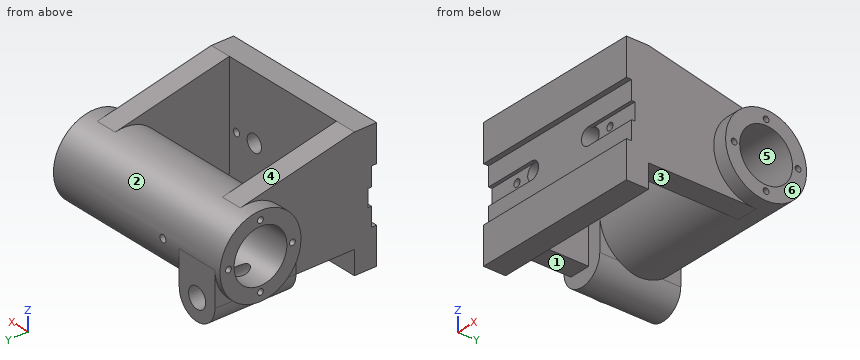
from build123d import *

# Parameters (mm, degrees)
SKETCH_2_R                   = 47.5
EXTRUDE_1_DEPTH              = 233
EXTRUDE_2_DEPTH              = 47.5
SKETCH_6_W                   = 200
SKETCH_6_H                   = 150
EXTRUDE_3_DEPTH              = 26
CUT_EXTRUDE_2_DEPTH          = 274.856257996
CUT_EXTRUDE_2_DEPTH_BACK     = 274.856257996
SKETCH_7_W                   = 64
SKETCH_7_H                   = 12
SKETCH_9_R                   = 10
CUT_EXTRUDE_3_DEPTH          = 20
SKETCH_11_W                  = 4.25
SKETCH_11_H                  = 20.001
HOLE_WIZARD_M10_1_AT_2_COUNT = 2
HOLE_WIZARD_M10_1_AT_2_PITCH = 130
CUT_EXTRUDE_START            = -60
SKETCH_12_W                  = 20
SKETCH_12_H                  = 8
CUT_EXTRUDE_4_DEPTH          = 60
EXTRUDE_6_DEPTH              = 25
RIB_8_REACH                  = 275.856
SKETCH_18_WALL_W             = 686.623983736
SKETCH_18_WALL_H             = 25
EXTRUDE_START                = -25
EXTRUDE_7_DEPTH              = 25
SKETCH_20_W                  = 25
SKETCH_20_H                  = 47.5
EXTRUDE_10_DEPTH             = 50
CUT_EXTRUDE_1_DEPTH          = 288.078386589
CUT_EXTRUDE_1_DEPTH_BACK     = 288.078386589
SKETCH_3_R                   = 31
HOLE_WIZARD_M8_1_AT_2_COUNT  = 2
HOLE_WIZARD_M8_1_AT_2_PITCH  = 53.033008589
HOLE_WIZARD_M8_1_AT_3_COUNT  = 2
HOLE_WIZARD_M8_1_AT_3_PITCH  = 75
HOLE_WIZARD_M8_1_AT_4_COUNT  = 2
HOLE_WIZARD_M8_1_AT_4_PITCH  = 53.033008589
SKETCH_27_W                  = 4.25
SKETCH_27_H                  = 47.5
SKETCH_16_R                  = 12
CUT_EXTRUDE_6_DEPTH          = 85


with BuildPart() as part:
    # Sketch 2 → Extrude 1 (new body)
    with BuildSketch(Plane(origin=(0, 0, 0), x_dir=(0, 0, -1), z_dir=(1, 0, 0))):
        Circle(SKETCH_2_R)
    extrude(amount=EXTRUDE_1_DEPTH)

    # Sketch 4 → Extrude 2 (add, symmetric)
    with BuildSketch(Plane(origin=(0, 0, 0), x_dir=(1, 0, 0), z_dir=(0, 1, 0))):
        with BuildLine():
            Line((7, 40), (7, 0))
            Line((7, 0), (57, 0))
            Line((57, 0), (57, 40))
            ThreePointArc((57, 40), (32, 65), (7, 40))
        make_face()
    extrude(amount=EXTRUDE_2_DEPTH, both=True)



with BuildPart() as body_2:
    # Sketch 6 → Extrude 3 (new body)
    with BuildSketch(Plane(origin=(0, -150, 0), x_dir=(1, 0, 0), z_dir=(0, 1, 0))):
        with Locations((116.5, 0)):
            Rectangle(SKETCH_6_W, SKETCH_6_H)
    extrude(amount=EXTRUDE_3_DEPTH)

    # Sketch 7 → Cut-Extrude 2 (cut, two sides: drawn at the far end of the back side and taken through both)
    with BuildSketch(Plane.ZY.offset(-16.5).offset(-CUT_EXTRUDE_2_DEPTH_BACK)):
        with Locations((0, -150)):
            Rectangle(SKETCH_7_W, SKETCH_7_H)
    extrude(amount=CUT_EXTRUDE_2_DEPTH + CUT_EXTRUDE_2_DEPTH_BACK, mode=Mode.SUBTRACT)

    # Sketch 9 → Cut-Extrude 3 (cut)
    with BuildSketch(Plane(origin=(0, -124, 0), x_dir=(1, 0, 0), z_dir=(0, 1, 0))):
        with Locations(Location((76.5, 0, 0), (0, 0, 270))):
            Circle(SKETCH_9_R)
        with Locations(Location((156.5, 0, 0), (0, 0, 270))):
            Circle(SKETCH_9_R)
    extrude(amount=-CUT_EXTRUDE_3_DEPTH, mode=Mode.SUBTRACT)

    # Sketch 11 → Hole Wizard M10 _1 (revolve, cut)
    with BuildSketch(Plane(origin=(181.5, -124, 0), x_dir=(0, 0, 1), z_dir=(1, 0, 0))):
        with Locations((2.125, 10.0005)):
            Rectangle(SKETCH_11_W, SKETCH_11_H)
    hole_wizard_m10_1 = revolve(axis=Axis((181.5, -117.65, 0), (0, -1, 0)), mode=Mode.SUBTRACT)

    # Hole Wizard M10 _1 at 2: Hole Wizard M10 _1 ×2
    with Locations(*[(-i * HOLE_WIZARD_M10_1_AT_2_PITCH, 0, 0) for i in range(1, HOLE_WIZARD_M10_1_AT_2_COUNT)]):
        add(hole_wizard_m10_1, mode=Mode.SUBTRACT)

    # Sketch 12 → Cut-Extrude 4 (cut)
    with BuildSketch(Plane.ZY.offset(-16.5).offset(CUT_EXTRUDE_START)):
        with Locations((0, -144)):
            Rectangle(SKETCH_12_W, SKETCH_12_H)
    cut_extrude_4 = extrude(amount=CUT_EXTRUDE_4_DEPTH, mode=Mode.SUBTRACT)

    # Mirror 1: Cut-Extrude 4 across plane
    add(cut_extrude_4.mirror(Plane.ZY.offset(-116.5)), mode=Mode.SUBTRACT)


with BuildPart() as part_1:
    add(part.part)

    add(body_2.part)  # Extrude 6 merges body 2
    # Sketch 13 → Extrude 6 (add)
    with BuildSketch(Plane.ZY.offset(-16.5)):
        with BuildLine():
            Line((-47.5, -124), (-35, -124))
            Line((-35, -124), (-35, -82.5))
            ThreePointArc((-35, -82.5), (-24.748737342, -57.751262658), (0, -47.5))
            Line((0, -47.5), (-47.5, -47.5))
            Line((-47.5, -47.5), (-47.5, -124))
        make_face()
    extrude(amount=-EXTRUDE_6_DEPTH)

    # Sketch 18 wall → Rib 8 (add, up to next)
    with BuildSketch(Plane(origin=(16.5, -57.048519027, 60.728115209), x_dir=(0, 0.978025903544, -0.208483409404), z_dir=(0, -0.208483409404, -0.978025903544)), mode=Mode.PRIVATE) as rib_8_sk1:
        with Locations((0, 12.5)):
            Rectangle(SKETCH_18_WALL_W, SKETCH_18_WALL_H)
    rib_8_tool1 = extrude(rib_8_sk1.sketch, amount=RIB_8_REACH, mode=Mode.PRIVATE) - part_1.part
    add(rib_8_tool1.solids().sort_by_distance((16.5, -57.048519027, 60.728115209))[0])

    # Sketch 19 → Extrude 7 (add)
    with BuildSketch(Plane(origin=(216.5, 0, 0), x_dir=(0, 0, -1), z_dir=(1, 0, 0)).offset(EXTRUDE_START)):
        with BuildLine():
            Line((47.5, -47.5), (0, -47.5))
            ThreePointArc((0, -47.5), (-36.92316815, -29.881928548), (-46.456230418, 9.902961947))
            Line((-46.456230418, 9.902961947), (-75, -124))
            Line((-75, -124), (47.5, -124))
            Line((47.5, -124), (47.5, -47.5))
        make_face()
    extrude(amount=EXTRUDE_7_DEPTH)

    # Sketch 20 → Extrude 10 (add)
    with BuildSketch(Plane(origin=(0, -47.5, 0), x_dir=(1, 0, 0), z_dir=(0, 1, 0))):
        with Locations((204, 23.75)):
            Rectangle(SKETCH_20_W, SKETCH_20_H)
    extrude(amount=EXTRUDE_10_DEPTH)

    # Sketch 3 → Cut-Extrude 1 (cut, two sides: drawn at the far end of the back side and taken through both)
    with BuildSketch(Plane.ZY.offset(-CUT_EXTRUDE_1_DEPTH_BACK)):
        Circle(SKETCH_3_R)
    extrude(amount=CUT_EXTRUDE_1_DEPTH + CUT_EXTRUDE_1_DEPTH_BACK, mode=Mode.SUBTRACT)

    # Sketch 25 → Hole Wizard M8 _1 (revolve, cut)
    with BuildSketch(Plane(origin=(0, 0, -37.5), x_dir=(0, 0, 1), z_dir=(0, 1, 0))):
        Polygon((0, 0), (0, 23), (3.4, 20.957073895), (3.4, 0), align=None)
    hole_wizard_m8_1 = revolve(axis=Axis((-6.35, 0, -37.5), (1, 0, 0)), mode=Mode.SUBTRACT)

    # Hole Wizard M8 _1 at 2: Hole Wizard M8 _1 ×2
    with Locations(*[Vector(0, 0.7071067811865476, 0.7071067811865476) * (i * HOLE_WIZARD_M8_1_AT_2_PITCH) for i in range(1, HOLE_WIZARD_M8_1_AT_2_COUNT)]):
        add(hole_wizard_m8_1, mode=Mode.SUBTRACT)

    # Hole Wizard M8 _1 at 3: Hole Wizard M8 _1 ×2
    with Locations(*[(0, 0, i * HOLE_WIZARD_M8_1_AT_3_PITCH) for i in range(1, HOLE_WIZARD_M8_1_AT_3_COUNT)]):
        add(hole_wizard_m8_1, mode=Mode.SUBTRACT)

    # Hole Wizard M8 _1 at 4: Hole Wizard M8 _1 ×2
    with Locations(*[Vector(0, -0.7071067811865476, 0.7071067811865476) * (i * HOLE_WIZARD_M8_1_AT_4_PITCH) for i in range(1, HOLE_WIZARD_M8_1_AT_4_COUNT)]):
        add(hole_wizard_m8_1, mode=Mode.SUBTRACT)

    # Mirror 6: Hole Wizard M8 _1 across plane
    add(hole_wizard_m8_1.mirror(Plane.ZY.offset(-116.5)), mode=Mode.SUBTRACT)

    # Mirror 6 copy 1 sketch → Mirror 6 copy 1 (revolve, cut)
    with BuildSketch(Plane(origin=(233, 37.5, 0), x_dir=(0, 0, 1), z_dir=(0, 1, 0))):
        Polygon((0, 0), (0, -23), (3.4, -20.957073895), (3.4, 0), align=None)
    revolve(axis=Axis((239.35, 37.5, 0), (1, 0, 0)), mode=Mode.SUBTRACT)

    # Mirror 6 copy 2 sketch → Mirror 6 copy 2 (revolve, cut)
    with BuildSketch(Plane(origin=(233, 0, 37.5), x_dir=(0, 0, 1), z_dir=(0, 1, 0))):
        Polygon((0, 0), (0, -23), (3.4, -20.957073895), (3.4, 0), align=None)
    revolve(axis=Axis((239.35, 0, 37.5), (1, 0, 0)), mode=Mode.SUBTRACT)

    # Mirror 6 copy 3 sketch → Mirror 6 copy 3 (revolve, cut)
    with BuildSketch(Plane(origin=(233, -37.5, 0), x_dir=(0, 0, 1), z_dir=(0, 1, 0))):
        Polygon((0, 0), (0, -23), (3.4, -20.957073895), (3.4, 0), align=None)
    revolve(axis=Axis((239.35, -37.5, 0), (1, 0, 0)), mode=Mode.SUBTRACT)

    # Sketch 27 → Hole Wizard M10 _1 2 (revolve, cut)
    with BuildSketch(Plane(origin=(80, 0, 0), x_dir=(0, 0, -1), z_dir=(1, 0, 0))):
        with Locations((2.125, 23.75)):
            Rectangle(SKETCH_27_W, SKETCH_27_H)
    revolve(axis=Axis((80, -6.35, 0), (0, 1, 0)), mode=Mode.SUBTRACT)

    # Sketch 16 → Cut-Extrude 6 (cut)
    with BuildSketch(Plane(origin=(0, 47.5, 0), x_dir=(1, 0, 0), z_dir=(0, 1, 0))):
        with Locations(Location((32, 40, 0), (0, 0, 270))):
            Circle(SKETCH_16_R)
    extrude(amount=-CUT_EXTRUDE_6_DEPTH, mode=Mode.SUBTRACT)


solid = part_1.part
Check sheet for the modelled part. Datum: model origin and axes. Units: mm. Face numbers are marked on the shaded views. A direction names the side the tool comes from. Round coordinates to 2 decimals unless told otherwise and drop trailing zeros. Write each loop counter-clockwise with the first axis right and the second up, starting at its lowest first coordinate (ties: lowest second). Pieces come first, ordered by that corner, then holes. Notation, with made-up numbers: (30.5, 39.5) -> (66.5, 39.5) arc R14 cw to (66.5, 60.5) -> close; hole circle Ø3 at (27.5, -19.5). An arc over 180 degrees is marked (long way). Answer as CSV lines item,"result". Start each with the question number.
1) Go/stop test with flat-tipped pins: P1, Ø6, axis at x = 129.5, z = -42, coming from the +Y side; P2, Ø5, axis at y = -88.5, z = 36, coming from the +X side; P3, Ø4, axis at x = 208.5, y = -5.5, coming from the +Z side; P4, Ø5, axis at y = -23, z = 58, coming from the +X side. Record where each tip stops, or that it passes through.
2) Section check C-C on x = 195.5. Enter the section's corners in (y, z), and give its area (3 significant figures).
3) Section check B-B on z = -55. Enter the section's corners in (x, y), and give its area (3 significant figures).
4) Tool access check on the marked faces 1, 2 and 3. Record the directions out of +Z, -Z, +X, -X, +Y, -Y that give a thin tool (end or side, any length) a straight path to the whole face; none if there is none.
5) Section check D-D on y = -109.5. Enter the section's corners in (x, z).
6) Release check for a two-part mould opening along Z. For the marked faces 4, 5 and 6 record: pulls with the +Z half, pulls with the -Z half, needs draft (parallel to the pull), parting line crosses it, or undercut.
7) Section check A-A on x = 125. Enter the section's corners in (y, z), and give its area (3 significant figures).
8) Material ranges on line 1 (X direction, y = -129, z = 0); line 2 (Y direction, x = 99, z = -1.5); line 3 (X direction, y = -109, z = -38), recorded low to high. Write a range as from..to.
Found:
1,P1,"stops at y = 27.12"
1,P2,"stops at x = 216.5"
1,P3,"stops at z = 50.17"
1,P4,"passes through"
2,outline,"(-150, -75) -> (-124, -75) -> (-124, -47.5) -> (2.5, -47.5) -> (2.5, -47.43) arc R47.5 ccw to (9.9, 46.46) -> (-124, 75) -> (-150, 75) -> (-150, 32) -> (-144, 32) -> (-144, 10) -> (-140, 10) -> (-140, -10) -> (-144, -10) -> (-144, -32) -> (-150, -32) -> close; hole circle Ø62 at (0, 0)"
2,area,"17,500 mm^2"
3,outline,"(12, -47.5) -> (52, -47.5) -> (52, 47.5) -> (12, 47.5) -> close; (16.5, -150) -> (216.5, -150) -> (216.5, -124) -> (16.5, -124) -> close"
3,area,"9,000 mm^2"
4,face 1,"-Z, +X, -X"
4,face 2,"none"
4,face 3,"-Z, +X, +Y"
5,outline,"(16.5, -47.5) -> (41.5, -47.5) -> (41.5, 71.91) -> (16.5, 71.91) -> close; (191.5, -47.5) -> (216.5, -47.5) -> (216.5, 71.91) -> (191.5, 71.91) -> close"
6,face 4,"pulls with the +Z half"
6,face 5,"undercut"
6,face 6,"needs draft"
7,outline,"(-150, -75) -> (-124, -75) -> (-124, 75) -> (-150, 75) -> (-150, 32) -> (-144, 32) -> (-144, -32) -> (-150, -32) -> close; circle Ø95 at (0, 0); hole circle Ø62 at (0, 0)"
7,area,"7,590 mm^2"
8,line 1,"x = 16.5..47.25, 55.75..66.5, 86.5..146.5, 166.5..177.25, 185.75..216.5"
8,line 2,"y = -144..-124, -47.48..-30.96, 30.96..47.48"
8,line 3,"x = 16.5..41.5, 191.5..216.5"
